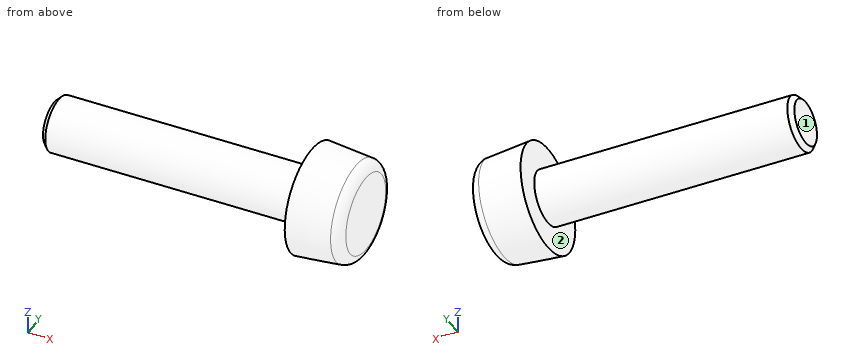
Autodesk Inventor part; units mm, degrees
ref_plane "AS_XY" through (12.5, 0, 0) normal (1, 0, 0) x (0, 0, -1)
ref_plane "AS_YZ" through (12.5, 0, 0) normal (0, 0, -1) x (0, 1, 0)
ref_plane "AS_ZX" through (12.5, 0, 0) normal (0, 1, 0) x (1, 0, 0)
sketch "Skizze_1" plane through (0, 0, 0) normal (0, 1, 0) x (-1, 0, 0)
  line L0 (-29, 0) -> (0, 0)
  line L1 (0, 0) -> (0, -2.067)
  line L2 (0, -2.067) -> (-0.433, -2.5)
  line L3 (-0.433, -2.5) -> (-24, -2.5)
  line L4 (-24, -2.5) -> (-24, -5)
  line L5 (-24, -5) -> (-28.0872, -4.6424)
  arc A0 (-29, -3.6462) -> (-28.0872, -4.6424) centre (-28, -3.6462) ccw
  line L6 (-29, -3.6462) -> (-29, 0)
  line L7 (-29, 0) -> (0, 0)
revolve "Revolution1" add sketch "Skizze_1" angle 360 about axis through (29, 0, 0) along (1, 0, 0)
thread "Thread1"
ref_plane "AS_XY" through (12.5, 0, 0) normal (1, 0, 0) x (0, 0, -1)
ref_plane "AS_YZ" through (12.5, 0, 0) normal (0, 0, -1) x (0, 1, 0)
ref_plane "AS_ZX" through (12.5, 0, 0) normal (0, 1, 0) x (1, 0, 0)
properties part number "305208-KOMP"
Geometry check sheet. Reference: the model listing, model coordinates, mm. Face numbers are marked on the shaded views. A direction names the side the tool comes from. Coordinates: 2 decimals unless noted, no trailing zeros. Loops run counter-clockwise (first coordinate to the right, second up) from the corner with the lowest first, then second, coordinate; pieces in that order, holes last. Notation, with made-up numbers: (38.25, 28) - (57.25, 28) arc R21 ccw to (57.25, 54) - close; hole circle Ø7 at (37, 71). An arc over 180 degrees is marked (long way). One line per item, written item: value. Start each with the question number.
(1) Cross-section at C-C on x = 19.5. Enter the section's corners in (y, z), plus the area to 3 significant figures.
(2) Cross-section at A-A on y = 0. Enter the section's corners in (x, z), plus the area to 3 significant figures.
(3) Tool access check on the marked faces 1 and 2. Record the directions out of +Z, -Z, +X, -X, +Y, -Y that give a thin tool (end or side, any length) a straight path to the whole face; none if there is none.
(4) Depth check by flat-ended pin: P1, Ø1.5, axis at y = 1, z = 3, coming from the -X side; P2, Ø6, axis at x = 14.5, z = -2, coming from the +Y side; P3, Ø1.5, axis at x = 6.5, y = 1.5, coming from the -Z side. Enter the tip coordinate at first touch or a pass-through.
(5) Material ranges on line 1 (X direction, y = -3.25, z = 0.75); line 2 (Y direction, x = 12.25, z = -1.25); line 3 (X direction, y = -3.25, z = 2.75), recorded low to high. Write a range as [from, to].
Results below:
1. outline: circle Ø5 at (0, 0)
1. area: 19.6 mm2
2. outline: (0, -2.07) - (0.43, -2.5) - (24, -2.5) - (24, -5) - (28.09, -4.64) arc R1 ccw to (29, -3.65) - (29, 3.65) arc R1 ccw to (28.09, 4.64) - (24, 5) - (24, 2.5) - (0.43, 2.5) - (0, 2.07) - close
2. area: 167 mm2
3. face 1: +Z, -Z, -X, +Y, -Y
3. face 2: -X
4. P1: stops at x = 0.35
4. P2: stops at y = 2.5
4. P3: stops at z = -2.38
5. line 1: x = [24, 29]
5. line 2: y = [-2.17, 2.17]
5. line 3: x = [24, 28.79]
